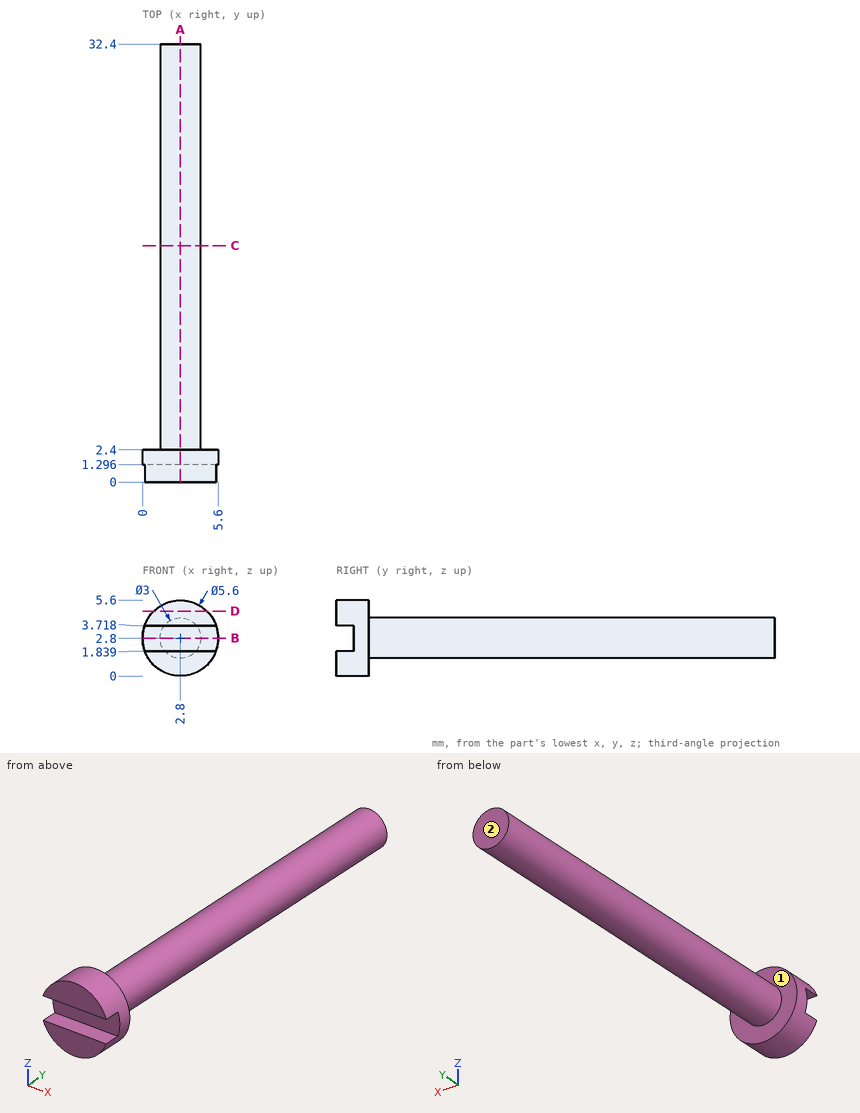
Here's the drawing with two shaded views (mm, measured from the low corner). I have some questions. A direction names the side the tool comes from. Give positions to 0.01 mm unless a question says otherwise; leave off trailing zeros. Order: outer loops, then holes, each group sorted by start corner. A loop starts at its lowest first (then second) coordinate and runs counter-clockwise, first axis right, second up. Notation, with made-up numbers: M 18,84.5 L 69,84.5 A23 ccw 69,110.5 Z; hole C -27.75,-11.75 d9. An arc over 180 degrees is marked long. Answer as a JSON object with one key per item and string values. Group by question number.
1) Please list where these lines run through material, in increasing order: L1, parallel to Y at x = 0.6, z = 3.6; L2, parallel to X at y = 30.5, z = 2.75; L3, parallel to Y at x = 2.95, z = 3.1. Write a range as [from, to].
2) Suppose I cut it at B-B, the plane z = 2.8. Write out the boundary of the cut face in (x, y).
3) Suppose I cut it at A-A, the plane x = 2.8. Write out the boundary of the cut face in (y, z).
4) I'm going to push flat-ended pins straight in: pin 1 Ø2 at (y, z) = (28.5, 4) entering from +X; pin 2 Ø0.6 at (x, y) = (1.5, 0.5) entering from +Z (1 decimal); pin 3 Ø2 at (x, y) = (1, 17) entering from -Z. Where does each tip first touch, or does it pass through?
5) On a 3-axis mill with a long thin cutter (end or side, diameter ignored), from which of +Z, -Z, +X, -X, +Y, -Y can I reach the whole of each face in a straight line? I mean the marked faces 1 and 2. Say none if no direction works.
6) Suppose I cut it at D-D, the plane z = 4.8. Write out the boundary of the cut face in (x, y).
7) Suppose I cut it at C-C, the plane y = 17.5. Write out the boundary of the cut face in (x, z).
Results found:
{
 "1": {"L1": "[1.3, 2.4]", "L2": "[1.3, 4.3]", "L3": "[1.3, 32.4]"},
 "2": {"outline": "M 0,1.3 L 5.6,1.3 L 5.6,2.4 L 4.3,2.4 L 4.3,32.4 L 1.3,32.4 L 1.3,2.4 L 0,2.4 Z"},
 "3": {"outline": "M 0,0 L 2.4,0 L 2.4,1.3 L 32.4,1.3 L 32.4,4.3 L 2.4,4.3 L 2.4,5.6 L 0,5.6 L 0,3.72 L 1.3,3.72 L 1.3,1.84 L 0,1.84 Z"},
 "4": {"pin 1": "x = 4.29", "pin 2": "z = 5.4", "pin 3": "z = 1.53"},
 "5": {"face 1": "+Y", "face 2": "+Z, -Z, +X, -X, +Y"},
 "6": {"outline": "M 0.84,0 L 4.76,0 L 4.76,2.4 L 0.84,2.4 Z"},
 "7": {"outline": "C 2.8,2.8 d3"}
}
